```python
from build123d import *

# Parameters (mm, degrees)
CYLINDER_FACE_R      = 5
BASE_CYLINDER_DEPTH  = 2.2
RECTANGULAR_THING_W  = 7.274105322
RECTANGULAR_THING_H  = 6.86202534
RECTANGULAR_DEPTH    = 8
SKETCH5_R            = 5
F_2ND_CYLINDER_DEPTH = 5
SKETCH6_R            = 4
F_3RD_CYLINDER_DEPTH = 6.3
SKETCH7_R            = 1.75
TOP_CYLINDER_DEPTH   = 5
SKETCH9_R            = 0.7
PRONGS_DEPTH         = 5
CUT_EXTRUDE1_DEPTH   = 1


with BuildPart() as part:
    # Cylinder Face → Base Cylinder (new body)
    with BuildSketch(Plane.XY):
        Circle(CYLINDER_FACE_R)
    extrude(amount=BASE_CYLINDER_DEPTH)

    # rectangular thing → rectangular (add)
    with BuildSketch(Plane.XY.offset(2.2)):
        Rectangle(RECTANGULAR_THING_W, RECTANGULAR_THING_H)
    extrude(amount=RECTANGULAR_DEPTH)

    # Sketch5 → 2nd Cylinder (add)
    with BuildSketch(Plane.XY.offset(10.2)):
        with Locations(Location((0, 0, 0), (0, 0, 223.330253175))):
            Circle(SKETCH5_R)
    extrude(amount=F_2ND_CYLINDER_DEPTH)

    # Sketch6 → 3rd Cylinder (add)
    with BuildSketch(Plane.XY.offset(15.2)):
        Circle(SKETCH6_R)
    extrude(amount=F_3RD_CYLINDER_DEPTH)

    # Sketch7 → Top Cylinder (add)
    with BuildSketch(Plane.XY.offset(21.5)):
        Circle(SKETCH7_R)
    extrude(amount=TOP_CYLINDER_DEPTH)

    # Sketch9 → Prongs? (add)
    with BuildSketch(Plane.XY.offset(21.5)):
        with Locations((0, 2.857502284)):
            Circle(SKETCH9_R)
        with Locations(Location((0, -2.857502284, 0), (0, 0, 180))):
            Circle(SKETCH9_R)
    extrude(amount=PRONGS_DEPTH)

    # Sketch10 → Cut-Extrude1 (cut)
    # profile 1 of 3: a face of its own
    with BuildSketch(Plane(origin=(0, 0, 0), x_dir=(-1, 0, 0), z_dir=(0, 0, -1))):
        Polygon((-3.458075012, 1.962360203), (-3.143972448, 1.962360203), (-3.143972448, -1.178665438), (-1.797818602, -1.178665438), (-1.797818602, -1.537639797), (-3.458075012, -1.537639797), align=None)
    # profile 2 of 3: a face of its own
    with BuildSketch(Plane(origin=(0, 0, 0), x_dir=(-1, 0, 0), z_dir=(0, 0, -1))):
        Polygon((-1.214485269, 1.962360203), (0.759873706, 1.962360203), (0.759873706, 1.603385844), (-0.900382705, 1.603385844), (-0.900382705, 0.526462767), (0.759873706, 0.526462767), (0.759873706, 0.167488408), (-0.900382705, 0.167488408), (-0.900382705, -1.178665438), (0.759873706, -1.178665438), (0.759873706, -1.537639797), (-1.214485269, -1.537639797), align=None)
    # profile 3 of 3: a face of its own
    with BuildSketch(Plane(origin=(0, 0, 0), x_dir=(-1, 0, 0), z_dir=(0, 0, -1))):
        with BuildLine():
            Line((1.388078834, -1.537639797), (1.388078834, 1.962360203))
            Line((1.388078834, 1.962360203), (2.094809603, 1.962360203))
            add(Edge.make_bspline(
                [(2.094809603, 1.962360203), (2.156278591, 1.961917633), (2.275036357, 1.96106259), (2.446648804, 1.955641199), (2.605432567, 1.946050733), (2.750865426, 1.932081207), (2.883346638, 1.914928173), (3.002505246, 1.893427769), (3.108957389, 1.868039598), (3.174426829, 1.846394148), (3.205386526, 1.83615828)],
                knots=[0, 0, 0, 0, 1.314313732, 2.53924729, 3.670748893, 4.714932338, 5.66265055, 6.526160246, 7.303039223, 8, 8, 8, 8], degree=3))
            add(Edge.make_bspline(
                [(3.205386526, 1.83615828), (3.245881265, 1.820727574), (3.325952458, 1.79021608), (3.43995958, 1.732659779), (3.547284943, 1.667446677), (3.648504088, 1.594490814), (3.741304915, 1.511726466), (3.829312811, 1.42266938), (3.908927535, 1.32408104), (3.981835831, 1.218006052), (4.047571491, 1.105694), (4.104710648, 0.987358891), (4.152164642, 0.863601683), (4.191557868, 0.734766535), (4.222604326, 0.600570157), (4.243786258, 0.460856291), (4.257757247, 0.316177102), (4.259161299, 0.218002638), (4.259873706, 0.16818953)],
                knots=[0, 0, 0, 0, 0.984719456, 1.947108742, 2.898477687, 3.838006223, 4.779231079, 5.722358779, 6.681677486, 7.655904652, 8.64651281, 9.637519902, 10.640069247, 11.656948941, 12.698408672, 13.768548281, 14.867775369, 16, 16, 16, 16], degree=3))
            add(Edge.make_bspline(
                [(4.259873706, 0.16818953), (4.259244738, 0.124928291), (4.258005292, 0.039677502), (4.246875976, -0.085963393), (4.230699656, -0.207876965), (4.205655458, -0.325482665), (4.175252945, -0.439810883), (4.136288794, -0.549643127), (4.091653297, -0.655986936), (4.039603419, -0.757404412), (3.982462034, -0.853487784), (3.921140291, -0.944063313), (3.855703595, -1.027838534), (3.785527962, -1.105067146), (3.711520246, -1.175632725), (3.633195915, -1.24012474), (3.550352865, -1.297281295), (3.463362142, -1.349348403), (3.369686013, -1.394768759), (3.267550146, -1.433198769), (3.156518968, -1.465045384), (3.036865011, -1.49161628), (2.908381534, -1.512693582), (2.770942568, -1.526819975), (2.624759278, -1.536372908), (2.524380013, -1.537209301), (2.472714251, -1.537639797)],
                knots=[0, 0, 0, 0, 1.105936401, 2.179363191, 3.223086493, 4.248585256, 5.251745608, 6.245858792, 7.225916811, 8.198733463, 9.158002045, 10.082870192, 10.993790845, 11.873723703, 12.748670949, 13.606408763, 14.465103618, 15.319838547, 16.196477973, 17.123216899, 18.106603292, 19.147568657, 20.255746949, 21.433717677, 22.679120308, 24, 24, 24, 24], degree=3))
            Line((2.472714251, -1.537639797), (1.388078834, -1.537639797))
        make_face()
        with BuildLine():
            Line((1.702181398, -1.178665438), (2.103924186, -1.178665438))
            add(Edge.make_bspline(
                [(2.103924186, -1.178665438), (2.161652557, -1.178417342), (2.272685356, -1.177940162), (2.432343353, -1.173752958), (2.578222749, -1.166911021), (2.710344259, -1.157335943), (2.828633283, -1.144667328), (2.933337033, -1.130542425), (3.024112291, -1.112944974), (3.079041728, -1.096994015), (3.104424988, -1.08962297)],
                knots=[0, 0, 0, 0, 1.375205317, 2.645023457, 3.804390687, 4.853969522, 5.800190428, 6.637939096, 7.370582563, 8, 8, 8, 8], degree=3))
            add(Edge.make_bspline(
                [(3.104424988, -1.08962297), (3.13637335, -1.078371412), (3.199506988, -1.056137039), (3.290388073, -1.015579378), (3.375145078, -0.967537308), (3.455255103, -0.914135034), (3.529581759, -0.853489032), (3.599005875, -0.786918043), (3.663387676, -0.714083268), (3.722061984, -0.635075106), (3.774570288, -0.550385311), (3.820041518, -0.460846477), (3.859893049, -0.367439667), (3.891171642, -0.268730508), (3.915687226, -0.16560145), (3.933051914, -0.058045236), (3.943866638, 0.053918045), (3.945128086, 0.13007017), (3.945771142, 0.168890652)],
                knots=[0, 0, 0, 0, 0.998632004, 1.973411704, 2.929992603, 3.868527914, 4.809262121, 5.754881198, 6.702106254, 7.672490631, 8.653608572, 9.636854334, 10.631411391, 11.644891563, 12.686317036, 13.754757253, 14.855430412, 16, 16, 16, 16], degree=3))
            add(Edge.make_bspline(
                [(3.945771142, 0.168890652), (3.945257854, 0.209824132), (3.944249497, 0.290238316), (3.931575186, 0.408229012), (3.913053631, 0.521709662), (3.886269945, 0.630687857), (3.852139066, 0.73537621), (3.809544424, 0.83519572), (3.760877805, 0.931200589), (3.702974468, 1.021174954), (3.639558875, 1.106268064), (3.569180995, 1.184222979), (3.492958957, 1.255217279), (3.411724107, 1.320356592), (3.323187008, 1.377020268), (3.229433317, 1.427706949), (3.129087646, 1.47072284), (3.05927495, 1.493601703), (3.023795981, 1.505228793)],
                knots=[0, 0, 0, 0, 1.122418816, 2.205001699, 3.251619955, 4.274784885, 5.280384055, 6.268708349, 7.249350384, 8.229342522, 9.199999885, 10.157847722, 11.105861043, 12.055065948, 13.010012805, 13.98527497, 14.976112212, 16, 16, 16, 16], degree=3))
            add(Edge.make_bspline(
                [(3.023795981, 1.505228793), (2.994444835, 1.51334522), (2.932036245, 1.530602973), (2.830196781, 1.549428346), (2.715581631, 1.566032845), (2.58768193, 1.580090884), (2.446643471, 1.590178205), (2.292357783, 1.59774952), (2.124758178, 1.602856152), (2.008575645, 1.60320486), (1.948275148, 1.603385844)],
                knots=[0, 0, 0, 0, 0.674548936, 1.434276114, 2.292660221, 3.240891867, 4.284742987, 5.42552168, 6.663806718, 8, 8, 8, 8], degree=3))
            Line((1.948275148, 1.603385844), (1.702181398, 1.603385844))
            Line((1.702181398, 1.603385844), (1.702181398, -1.178665438))
        make_face(mode=Mode.SUBTRACT)
    extrude(amount=-CUT_EXTRUDE1_DEPTH, mode=Mode.SUBTRACT)


solid = part.part
```
The listing builds one solid part. Answer for the finished solid, in the listing's coordinates (mm). A direction names the side the tool comes from. Give positions to 0.01 mm unless a question says otherwise; leave off trailing zeros. Order: outer loops, then holes, each group sorted by start corner. A loop starts at its lowest first (then second) coordinate and runs counter-clockwise, first axis right, second up. Notation, with made-up numbers: (51, 85.25) -> (99, 85.25) arc R31 ccw to (99, 109.25) -> close; hole circle Ø10 at (-26.5, 22.5). An arc over 180 degrees is marked (long way). One line per item, written item: value.
1) Find section C-C, the plane x = 2.75. Determine the outline of the cut face in (y, z).
Reported:
outline: (-4.18, 0) -> (-1.54, 0) -> (-1.54, 1) -> (-1.18, 1) -> (-1.18, 0) -> (4.18, 0) -> (4.18, 2.2) -> (3.43, 2.2) -> (3.43, 10.2) -> (4.18, 10.2) -> (4.18, 15.2) -> (2.9, 15.2) -> (2.9, 21.5) -> (-2.9, 21.5) -> (-2.9, 15.2) -> (-4.18, 15.2) -> (-4.18, 10.2) -> (-3.43, 10.2) -> (-3.43, 2.2) -> (-4.18, 2.2) -> close
2) Find section B-B, the plane z = 14.25. Determine the outline of the cut face in (x, y), plus the area to 3 significant figures.
Reported:
outline: circle Ø10 at (0, 0)
area: 78.5 mm^2
3) Find the intervals of material crossed by line 1 (Y direction, x = 0, z = 22.75); line 2 (Z direction, x = 3, y = -3.75); line 3 (Z direction, x = 0, y = -1.5), in increasing order.
Reported:
line 1: y = -3.56 to -2.16, -1.75 to 1.75, 2.16 to 3.56
line 2: z = 0 to 2.2, 10.2 to 15.2
line 3: z = 1 to 26.5
4) Flat-ended cylindrical pins translate along their axes: P1, Ø1.1, axis at y = 1, z = 0.5, coming from the +X side; P2, Ø5, axis at y = -3, z = 9.5, coming from the -X side; P3, Ø2, axis at x = 0.5, z = 7.5, coming from the -Y side. Find the tip coordinate at first contact, or state that the pin passes through.
Reported:
P1: stops at x = 4.98
P2: stops at x = -4.96
P3: stops at y = -3.43
5) Find section D-D, the plane y = -2.5. Determine the outline of the cut face in (x, z).
Reported:
outline: (-4.33, 0) -> (4.33, 0) -> (4.33, 2.2) -> (3.64, 2.2) -> (3.64, 10.2) -> (4.33, 10.2) -> (4.33, 15.2) -> (3.12, 15.2) -> (3.12, 21.5) -> (0.6, 21.5) -> (0.6, 26.5) -> (-0.6, 26.5) -> (-0.6, 21.5) -> (-3.12, 21.5) -> (-3.12, 15.2) -> (-4.33, 15.2) -> (-4.33, 10.2) -> (-3.64, 10.2) -> (-3.64, 2.2) -> (-4.33, 2.2) -> close
6) Determine the mould class of faces 1 (the flat face through (0, -3.431, 6)), 2 (the flat face through (0.9, 1.1, 0.5)), 3 (the flat face through (0.1, 0.526, 0.5)), 4 (the cylindrical face through (-0.867, -3.905, 18.306)) for opening direction X: pulls with the +X half, pulls with the -X half, needs draft (parallel to the pull), parting line crosses it, or undercut.
Reported:
face 1: needs draft
face 2: undercut
face 3: undercut
face 4: parting line crosses it
7) Find section A-A, the plane y = 4.25. Determine the outline of the cut face in (x, z), plus the area to 3 significant figures.
Reported:
outline: (-2.63, 0) -> (2.63, 0) -> (2.63, 2.2) -> (-2.63, 2.2) -> close; (-2.63, 10.2) -> (2.63, 10.2) -> (2.63, 15.2) -> (-2.63, 15.2) -> close
area: 37.9 mm^2
8) A tool of negligible diameter and unlimited length cuts with its end or side. For faces 5 (the flat face through (0.2, -1.538, 0.5)), 6 (the flat face through (4, 0, 2.2)), 7 (the flat face through (-4, 0, 10.2)), 8 (the flat face through (0, 3.431, 6)), from which of +Z, -Z, +X, -X, +Y, -Y can it reach the whole face along a straight path? Write none if from no direction.
Reported:
face 5: -Z
face 6: +X, +Y, -Y
face 7: -X, +Y, -Y
face 8: +X, -X, +Y
